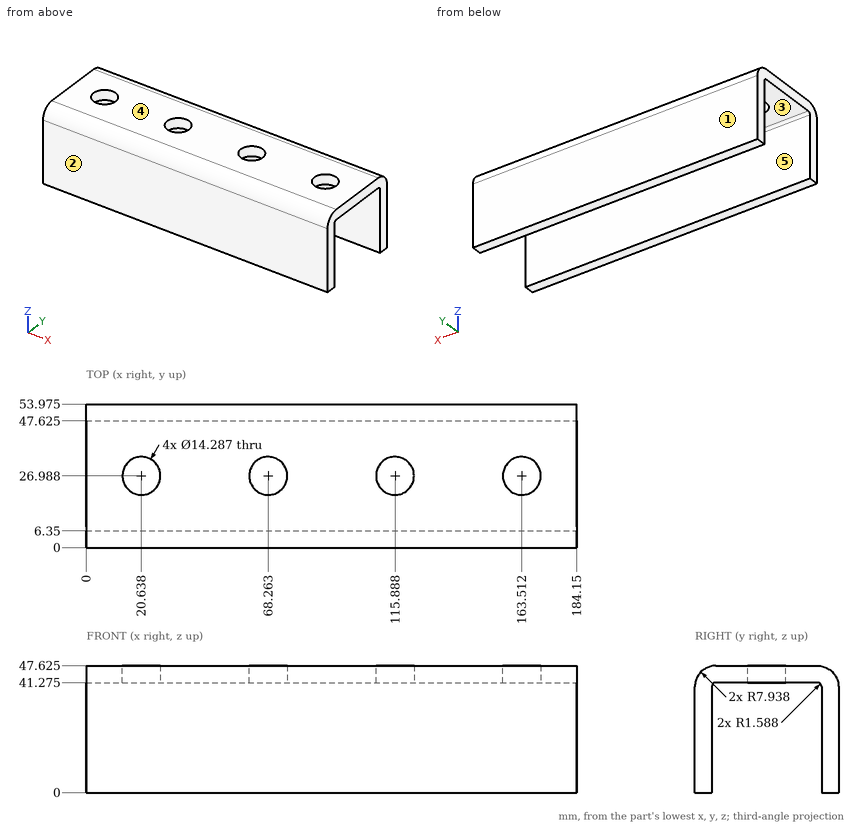
Could you check a few things on this drawing? It's one solid part, dimensions in mm from its lowest x, y, z. A direction names the side the tool comes from. Round coordinates to 2 decimals unless told otherwise and drop trailing zeros. Write each question's results on one line, items separated by ' | '. Start each with the question number.
(1) Thinking about a two-plate mould opening in Y: for the marked faces 1, 2 and 3, which applies, pulls with the +Y half, pulls with the -Y half, needs draft (parallel to the pull), parting line crosses it, or undercut?
(2) Will these pins go through, and if not, where does the flat tip stop? P1, Ø11.5, axis at x = 67.5, y = 36.5, coming from the -Z side (1 decimal); P2, Ø10, axis at x = 144, y = 47.5, coming from the -Z side.
(3) On a 3-axis mill with a long thin cutter (end or side, diameter ignored), from which of +Z, -Z, +X, -X, +Y, -Y can I reach the whole of each face in a straight line? I mean the marked faces 4 and 5. Say none if no direction works.
(4) If I drill on probe 1 along Z at (x, y) = (39.5, 40) (1 decimal); probe 2 along Z at (x, y) = (96.5, 4.5); probe 3 along Y at (x, z) = (150.5, 41.5) (1 decimal), over which ranges is the centre line in solid material (lowest first)? Write a range as from..to.
Solved:
1) face 1: pulls with the +Y half | face 2: pulls with the -Y half | face 3: undercut
2) P1: stops at z = 41.3 | P2: stops at z = 0
3) face 4: +Z, +X, -X, +Y, -Y | face 5: -Z, +X, -X
4) probe 1: z = 41.3..47.6 | probe 2: z = 0..46.84 | probe 3: y = 0.2..53.8
